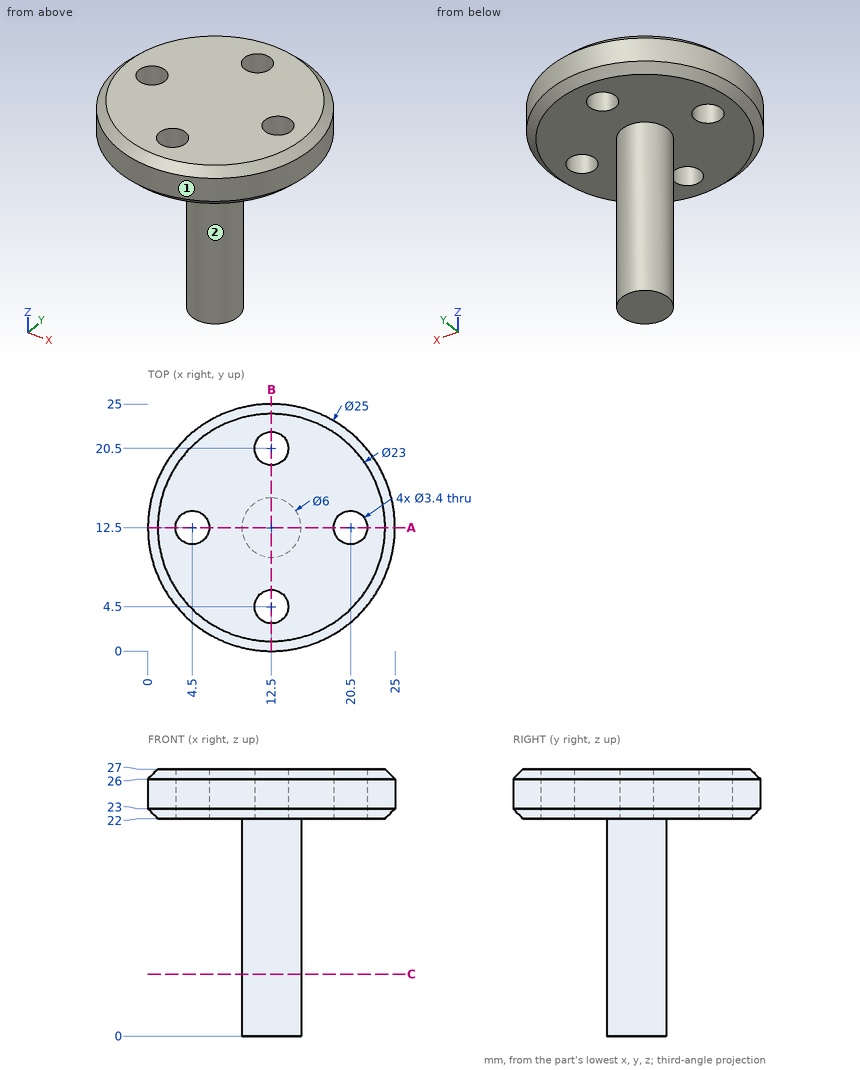
Study the drawing (mm; zero at the part's minimum x, y, z) and answer. A direction names the side the tool comes from. Coordinates: 2 decimals unless noted, no trailing zeros. Write each loop counter-clockwise with the first axis right and the second up, starting at its lowest first coordinate (ties: lowest second). Pieces come first, ordered by that corner, then holes. Notation, with made-up numbers: M 28.25,4.5 L 51.25,4.5 A21 ccw 51.25,27.5 Z; hole C 33,25.25 d3. An arc over 180 degrees is marked long. Write each question's results on one line, items separated by ' | '.
Item 1: The part is cut by section C-C on z = 6.25. Determine the outline of the cut face in (x, y).
Answer below:
outline: C 12.5,12.5 d6
Item 2: Which of the six approach directions +Z, -Z, +X, -X, +Y, -Y give full straight-line access (tool end or side, diameter ignored) to the marked faces 1 and 2?
Answer below:
face 1: +Z, -Z | face 2: -Z
Item 3: The part is cut by section A-A on y = 12.5. Determine the outline of the cut face in (x, z).
Answer below:
outline: M 0,23 L 1,22 L 2.8,22 L 2.8,27 L 1,27 L 0,26 Z; M 6.2,22 L 9.5,22 L 9.5,0 L 15.5,0 L 15.5,22 L 18.8,22 L 18.8,27 L 6.2,27 Z; M 22.2,22 L 24,22 L 25,23 L 25,26 L 24,27 L 22.2,27 Z
Item 4: Consider probe 1 along Y at (x, z) = (12.5, 23.45); probe 2 along Z at (x, y) = (10.25, 16.5). Determine where each line is inside the solid, lowest interval first. Write a range as [from, to].
Answer below:
probe 1: [0, 2.8], [6.2, 18.8], [22.2, 25] | probe 2: [22, 27]
Item 5: Given P1, Ø1.5, axis at x = 5, y = 22.5, coming from the +Z side; P2, Ø3, axis at y = 13, z = 16.5, coming from the +X side; P3, Ø4, axis at x = 4.5, y = 12.5, coming from the -Z side, each flat-ended and moving along its own axis, determine where each tip first touches the part or whether it passes through.
Answer below:
P1: z = 26.75 | P2: x = 15.5 | P3: z = 22
